Geometry: final body of the model. Coordinates: model frame, mm. A direction names the side the tool comes from. Coordinates: 2 decimals unless noted, no trailing zeros. Write each loop counter-clockwise with the first axis right and the second up, starting at its lowest first coordinate (ties: lowest second). Pieces come first, ordered by that corner, then holes. Notation, with made-up numbers: (-38.75, 50.25) -> (3.25, 50.25) arc R37 ccw to (3.25, 88.25) -> close; hole circle Ø11 at (42, 39). An arc over 180 degrees is marked (long way). Answer as a JSON object with one key per item and string values. Group by question number.
```python
from build123d import *

# Parameters (mm, degrees)
SKETCH1_R           = 2.1
BOSS_EXTRUDE1_DEPTH = 3
SKETCH2_W           = 40
SKETCH2_H           = 3.25
BOSS_EXTRUDE2_DEPTH = 13
SKETCH3_R           = 2.1
CUT_EXTRUDE1_DEPTH  = 15
FILLET1_R           = 5
BOSS_EXTRUDE3_DEPTH = 3
BOSS_EXTRUDE4_DEPTH = 3
FILLET4_R           = 6
SKETCH7_W           = 3.5
SKETCH7_H           = 9.863589554
CUT_EXTRUDE2_DEPTH  = 10
SKETCH8_W           = 3
SKETCH8_H           = 1.69787118
CUT_EXTRUDE3_DEPTH  = 10


with BuildPart() as part:
    # Sketch1 → Boss-Extrude1 (new body)
    with BuildSketch(Plane(origin=(0, 0, 0), x_dir=(1, 0, 0), z_dir=(0, 1, 0))):
        with BuildLine():
            Line((0, 20), (32, 20))
            ThreePointArc((32, 20), (34.828427125, 18.828427125), (36, 16))
            Line((36, 16), (36, -16))
            Line((36, -16), (36, -23.351584796))
            Line((36, -23.351584796), (-4, -23.351584796))
            Line((-4, -23.351584796), (-4, -16))
            Line((-4, -16), (-4, 16))
            ThreePointArc((-4, 16), (-2.828427125, 18.828427125), (0, 20))
        make_face()
        with Locations(Location((0, 16, 0), (0, 0, 270))):
            Circle(SKETCH1_R, mode=Mode.SUBTRACT)
        with Locations(Location((0, -16, 0), (0, 0, 270))):
            Circle(SKETCH1_R, mode=Mode.SUBTRACT)
        with Locations(Location((32, 16, 0), (0, 0, 270))):
            Circle(SKETCH1_R, mode=Mode.SUBTRACT)
        with Locations(Location((32, -16, 0), (0, 0, 270))):
            Circle(SKETCH1_R, mode=Mode.SUBTRACT)
        with BuildLine():
            Line((0, 12), (0, -12))
            ThreePointArc((0, -12), (2.828427125, -13.171572875), (4, -16))
            Line((4, -16), (28, -16))
            ThreePointArc((28, -16), (29.171572875, -13.171572875), (32, -12))
            Line((32, -12), (32, 12))
            ThreePointArc((32, 12), (29.171572875, 13.171572875), (28, 16))
            Line((28, 16), (4, 16))
            ThreePointArc((4, 16), (2.828427125, 13.171572875), (0, 12))
        make_face(mode=Mode.SUBTRACT)
    extrude(amount=BOSS_EXTRUDE1_DEPTH)

    # Sketch2 → Boss-Extrude2 (add)
    with BuildSketch(Plane(origin=(0, 3, 0), x_dir=(1, 0, 0), z_dir=(0, 1, 0))):
        with Locations((16, -21.726584796)):
            Rectangle(SKETCH2_W, SKETCH2_H)
    extrude(amount=BOSS_EXTRUDE2_DEPTH)

    # Sketch3 → Cut-Extrude1 (cut)
    with BuildSketch(Plane(origin=(0, 0, 20.101584796), x_dir=(-1, 0, 0), z_dir=(0, 0, -1))):
        with Locations((-0.000616802, 9.396216068)):
            Circle(SKETCH3_R)
        with Locations((-31.999383198, 9.396216068)):
            Circle(SKETCH3_R)
    extrude(amount=-CUT_EXTRUDE1_DEPTH, mode=Mode.SUBTRACT)

    # Fillet1
    fillet1_edges = [part.edges().sort_by_distance(p)[0] for p in [
        (-4, 16, 21.726584796),
        (36, 16, 21.726584796),
    ]]
    fillet(fillet1_edges, radius=FILLET1_R)

    # Sketch4 → Boss-Extrude3 (add)
    with BuildSketch(Plane(origin=(36, 0, 0), x_dir=(0, 0, -1), z_dir=(1, 0, 0))):
        Polygon((-20.101584796, 11), (12, 3.88638768), (12, 0), (-23.351584796, 0), (-23.351584796, 11), align=None)
    extrude(amount=BOSS_EXTRUDE3_DEPTH)

    # Sketch5 → Boss-Extrude4 (add)
    with BuildSketch(Plane.ZY.offset(4)):
        Polygon((20.101584796, 11), (23.351584796, 11), (23.351584796, 0), (-12, 0), (-12, 3.88638768), align=None)
    extrude(amount=BOSS_EXTRUDE4_DEPTH)

    # Fillet4
    # the kernel refuses this fillet: 6 mm, written as the material it adds along each edge
    with BuildSketch(Plane(origin=(36, 11, 23.351584796), x_dir=(1, 0, 0), z_dir=(0, 0, -1))) as fillet4_piece_1:
        with BuildLine():
            CenterArc((4.3125, -5.854685623), FILLET4_R, 102.635625093, 45.207166298)
            ThreePointArc((-0.767045455, -2.661220738), (-0.195586783, -1.384779274), (0, 0))
            Line((0, 0), (3, 0))
        make_face()
    extrude(amount=3.25)
    with BuildSketch(Plane(origin=(-4, 11, 20.101584796), x_dir=(0.2769558547034986, 0.9608826434822593, 0), z_dir=(0, 0, 1))) as fillet4_piece_2:
        with BuildLine():
            CenterArc((4.431293675, 5.765295861), FILLET4_R, 208.714229398, 45.207166298)
            Line((-0.830867564, 2.88264793), (0, 0))
            ThreePointArc((0, 0), (1.384779274, 0.195586783), (2.769558547, 0))
        make_face()
    extrude(amount=3.25)

    # Sketch7 → Cut-Extrude2 (cut)
    with BuildSketch(Plane(origin=(0, 3, 0), x_dir=(1, 0, 0), z_dir=(0, 1, 0))):
        with Locations((-5.25, 15.233923597)):
            Rectangle(SKETCH7_W, SKETCH7_H)
        with Locations((37.25, 15.233923597)):
            Rectangle(SKETCH7_W, SKETCH7_H)
    extrude(amount=-CUT_EXTRUDE2_DEPTH, mode=Mode.SUBTRACT)

    # Sketch8 → Cut-Extrude3 (cut)
    with BuildSketch(Plane(origin=(0, 3, 0), x_dir=(-1, 0, 0), z_dir=(0, -1, 0))):
        with Locations((5.5, 11.15106441)):
            Rectangle(SKETCH8_W, SKETCH8_H)
        with Locations((-37.5, 11.15106441)):
            Rectangle(SKETCH8_W, SKETCH8_H)
    extrude(amount=-CUT_EXTRUDE3_DEPTH, mode=Mode.SUBTRACT)


solid = part.part
```
Item 1: Section B-B on z = 8.5. Output: boundary loops of the cut face in (x, y).
Item 2: Section D-D on y = 12.25. Output: boundary loops of the cut face in (x, z), then the cut area to 3 significant figures.
Item 3: Set-up query: faces 1 (the cylindrical face through (29.203, 1.479, -13.141)), 2 (the flat face through (35.5, 2, -14)), 3 (the flat face through (-5.479, 7.584, 4.687)). Return all of +Z, -Z, +X, -X, +Y, -Y with unobstructed straight access to the full face (end or side cutting, diameter ignored); none if empty.
Item 4: Contact query for flat-ended pins moving along their axis: pin 1 (8 mm diameter, centred on x = 18.5, z = 14.5, fed in from +Y); pin 2 (6.5 mm diameter, centred on x = 32, y = 9.4, fed in from -Z); pin 3 (1.8 mm diameter, centred on x = 36.5, y = 3, fed in from -Z). Output: stop coordinate, or through.
Item 5: Ray query, L1, parallel to X at y = 3.25, z = 6.5; L2, parallel to X at y = 2.5, z = 2; L3, parallel to Z at x = 1, y = 15. Return the intervals inside material, ascending. Write a range as [from, to].
Item 6: Section A-A on x = 12.5. Output: boundary loops of the cut face in (y, z), then the cut area to 3 significant figures.
Item 7: Section C-C on z = 14.5. Output: boundary loops of the cut face in (x, y), then the cut area to 3 significant figures.
Answer sheet:
{
 "1": {"outline": "(-7, 0) -> (0, 0) -> (0, 3) -> (-4, 3) -> (-4, 8.43) -> (-7, 8.43) -> close; (32, 0) -> (39, 0) -> (39, 8.43) -> (36, 8.43) -> (36, 3) -> (32, 3) -> close"},
 "2": {"outline": "(-4.47, 20.1) -> (36.47, 20.1) -> (36.47, 23.35) -> (-4.47, 23.35) -> close", "area": "133 mm^2"},
 "3": {"face 1": "+Y, -Y", "face 2": "-Z, +X, +Y, -Y", "face 3": "-Z, +X, -X, +Y"},
 "4": {"pin 1": "stops at y = 3", "pin 2": "stops at z = 20.1", "pin 3": "stops at z = -10.3"},
 "5": {"L1": "x = [-7, -4], [36, 39]", "L2": "x = [-7, 0], [32, 39]", "L3": "z = [20.1, 23.35]"},
 "6": {"outline": "(0, -20) -> (3, -20) -> (3, -16) -> (0, -16) -> close; (0, 16) -> (3, 16) -> (3, 20.1) -> (16, 20.1) -> (16, 23.35) -> (0, 23.35) -> close", "area": "76.3 mm^2"},
 "7": {"outline": "(-7, 0) -> (-1.47, 0) -> (-1.47, 3) -> (-4, 3) -> (-4, 9.76) -> (-7, 9.76) -> close; (1.47, 0) -> (3.71, 0) -> (3.71, 3) -> (1.47, 3) -> close; (28.29, 0) -> (30.53, 0) -> (30.53, 3) -> (28.29, 3) -> close; (33.47, 0) -> (39, 0) -> (39, 9.76) -> (36, 9.76) -> (36, 3) -> (33.47, 3) -> close", "area": "87.2 mm^2"}
}
